from build123d import *

# Parameters (mm, degrees)
SKETCH1_W           = 210
SKETCH1_H           = 20
BOSS_EXTRUDE1_DEPTH = 8
SKETCH2_R           = 4
CUT_EXTRUDE1_DEPTH  = 10
LPATTERN1_COUNT     = 8
LPATTERN1_PITCH     = 20
SKETCH4_W           = 80
SKETCH4_H           = 20
CUT_EXTRUDE2_DEPTH  = 10


with BuildPart() as part:
    # Sketch1 → Boss-Extrude1 (new body)
    with BuildSketch(Plane(origin=(0, 0, 0), x_dir=(1, 0, 0), z_dir=(0, 1, 0))):
        with Locations((105, 10)):
            Rectangle(SKETCH1_W, SKETCH1_H)
    extrude(amount=BOSS_EXTRUDE1_DEPTH)

    # Sketch2 → Cut-Extrude1 (cut)
    with BuildSketch(Plane(origin=(0, 8, 0), x_dir=(1, 0, 0), z_dir=(0, 1, 0))):
        with Locations(Location((195, 10, 0), (0, 0, 270))):
            Circle(SKETCH2_R)
    cut_extrude1 = extrude(amount=-CUT_EXTRUDE1_DEPTH, mode=Mode.SUBTRACT)

    # LPattern1: Cut-Extrude1 ×8
    with Locations(*[(-i * LPATTERN1_PITCH, 0, 0) for i in range(1, LPATTERN1_COUNT)]):
        add(cut_extrude1, mode=Mode.SUBTRACT)

    # Sketch4 → Cut-Extrude2 (cut)
    with BuildSketch(Plane(origin=(0, 0, 0), x_dir=(1, 0, 0), z_dir=(0, 1, 0))):
        with Locations((-10, 10)):
            Rectangle(SKETCH4_W, SKETCH4_H)
    extrude(amount=CUT_EXTRUDE2_DEPTH, mode=Mode.SUBTRACT)


solid = part.part
Read the model definition and answer for the solid it produces. Units are mm, in the model's axes. Coordinates: 2 decimals unless noted, no trailing zeros. Order: outer loops, then holes, each group sorted by start corner. A loop starts at its lowest first (then second) coordinate and runs counter-clockwise, first axis right, second up. Notation, with made-up numbers: M 1.5,5 L 39.5,5 A4 cw 39.5,11 Z; hole C 14,16 d2. An arc over 180 degrees is marked long. Put each result on its own line as item: value. Start each with the question number.
Item 1: Consider probe 1 along Z at (x, y) = (58.5, 1); probe 2 along Z at (x, y) = (152.5, 7.5). Determine where each line is inside the solid, lowest interval first. Write a range as [from, to].
Item 2: Section A-A, the plane x = 95 is taken. Determine the outline of the cut face in (y, z), plus the area to 3 significant figures.
Item 3: The mould has two halves that part along Z. Classify faces 1 (the face through (119, 4, 0)), 2 (the face through (119, 4, -20)), 3 (the face through (51.095, 4.056, -10.867)): +Z half, -Z half, draft (parallel to the pull), parting line (faces both ways), or undercut.
Item 4: Section B-B, the plane y = 3 is taken. Count the separate pieces of the cut face and the enclosed holes in it, plus the area to 3 significant figures.
Item 5: Section D-D, the plane x = 192.5 is taken. Determine the outline of the cut face in (y, z).
Computed:
1. probe 1: z = [-20, -11.94], [-8.06, 0]
1. probe 2: z = [-20, -13.12], [-6.88, 0]
2. outline: M 0,-20 L 8,-20 L 8,-14 L 0,-14 Z; M 0,-6 L 8,-6 L 8,0 L 0,0 Z
2. area: 96.0 mm2
3. face 1: +Z half
3. face 2: -Z half
3. face 3: undercut
4. separate pieces: 1
4. enclosed holes: 8
4. area: 3,200 mm2
5. outline: M 0,-20 L 8,-20 L 8,-13.12 L 0,-13.12 Z; M 0,-6.88 L 8,-6.88 L 8,0 L 0,0 Z
